from build123d import *

# Parameters (mm, degrees)
EXTRUDE_1_DEPTH     = 3
SKETCH_2_W          = 10.5
SKETCH_2_H          = 3.5
CUT_EXTRUDE_1_DEPTH = 150.258104234


with BuildPart() as part:
    # Эскиз1 → Бобышка-Вытянуть1 (new body)
    with BuildSketch(Plane(origin=(0, 0, 0), x_dir=(1, 0, 0), z_dir=(0, 1, 0))):
        with BuildLine():
            Line((-135, -31.788922156), (-138, -31.788922156))
            Line((-138, -31.788922156), (-138, -21.788922156))
            Line((-138, -21.788922156), (-135, -21.788922156))
            Line((-135, -21.788922156), (-135, -16.788922156))
            Line((-135, -16.788922156), (-138, -16.788922156))
            Line((-138, -16.788922156), (-138, -6.788922156))
            Line((-138, -6.788922156), (-135, -6.788922156))
            Line((-135, -6.788922156), (-135, 3.211077844))
            Line((-135, 3.211077844), (-125, 3.211077844))
            Line((-125, 3.211077844), (75, 3.211077844))
            Line((75, 3.211077844), (85, 3.211077844))
            Line((85, 3.211077844), (85, -6.788922156))
            Line((85, -6.788922156), (88, -6.788922156))
            Line((88, -6.788922156), (88, -16.788922156))
            Line((88, -16.788922156), (85, -16.788922156))
            Line((85, -16.788922156), (85, -21.788922156))
            Line((85, -21.788922156), (88, -21.788922156))
            Line((88, -21.788922156), (88, -31.788922156))
            Line((88, -31.788922156), (85, -31.788922156))
            Line((85, -31.788922156), (85, -36.788922156))
            Line((85, -36.788922156), (88, -36.788922156))
            Line((88, -36.788922156), (88, -46.788922156))
            Line((88, -46.788922156), (85, -46.788922156))
            Line((85, -46.788922156), (85, -56.788922156))
            Line((85, -56.788922156), (55, -56.788922156))
            Line((55, -56.788922156), (55, -26.788922156))
            ThreePointArc((55, -26.788922156), (52.071067812, -19.717854344), (45, -16.788922156))
            Line((45, -16.788922156), (-95, -16.788922156))
            ThreePointArc((-95, -16.788922156), (-102.071067812, -19.717854344), (-105, -26.788922156))
            Line((-105, -26.788922156), (-105, -56.788922156))
            Line((-105, -56.788922156), (-135, -56.788922156))
            Line((-135, -56.788922156), (-135, -46.788922156))
            Line((-135, -46.788922156), (-138, -46.788922156))
            Line((-138, -46.788922156), (-138, -36.788922156))
            Line((-138, -36.788922156), (-135, -36.788922156))
            Line((-135, -36.788922156), (-135, -31.788922156))
        make_face()
    extrude(amount=EXTRUDE_1_DEPTH)

    # Эскиз2 → Вырез-Вытянуть1 (cut, through all)
    with BuildSketch(Plane(origin=(0, 0, 0), x_dir=(1, 0, 0), z_dir=(0, 1, 0))):
        with Locations((-115, -10.788922156)):
            Rectangle(SKETCH_2_W, SKETCH_2_H)
        with Locations((-95, -10.788922156)):
            Rectangle(SKETCH_2_W, SKETCH_2_H)
        with Locations((-75, -10.788922156)):
            Rectangle(SKETCH_2_W, SKETCH_2_H)
        with Locations((-55, -10.788922156)):
            Rectangle(SKETCH_2_W, SKETCH_2_H)
        with Locations((-35, -10.788922156)):
            Rectangle(SKETCH_2_W, SKETCH_2_H)
        with Locations((-15, -10.788922156)):
            Rectangle(SKETCH_2_W, SKETCH_2_H)
        with Locations((5, -10.788922156)):
            Rectangle(SKETCH_2_W, SKETCH_2_H)
        with Locations((25, -10.788922156)):
            Rectangle(SKETCH_2_W, SKETCH_2_H)
        with Locations((45, -10.788922156)):
            Rectangle(SKETCH_2_W, SKETCH_2_H)
        with Locations((65, -10.788922156)):
            Rectangle(SKETCH_2_W, SKETCH_2_H)
    extrude(amount=CUT_EXTRUDE_1_DEPTH, mode=Mode.SUBTRACT)


solid = part.part
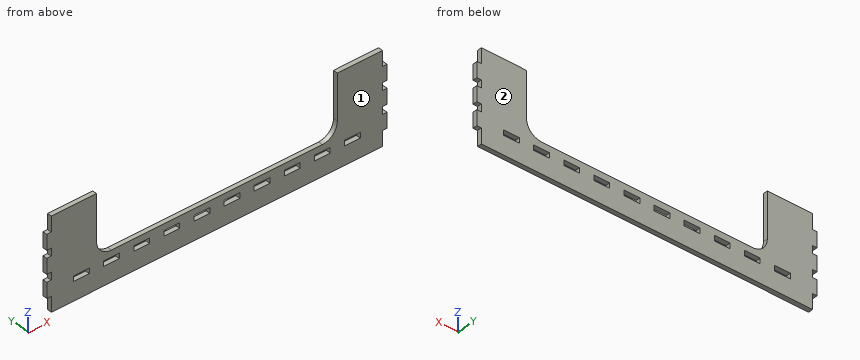
Work out the finished part from the listing and answer in its coordinate system (mm). Face numbers are marked on the shaded views. Give positions to 0.01 mm unless a question says otherwise; leave off trailing zeros. Loops run counter-clockwise (first coordinate to the right, second up) from the corner with the lowest first, then second, coordinate; pieces in that order, holes last. Notation, with made-up numbers: (47, 51) -> (72, 51) arc R25 cw to (72, 74) -> close; hole circle Ø5 at (24, 15). An arc over 180 degrees is marked (long way). Use a Markdown table: item, result. Add a question column.
1. Find the intervals of material crossed by probe 1 along Z at (x, y) = (5.5, 2.1); probe 2 along Z at (x, y) = (62, 0.45); probe 3 along X at (y, z) = (2.25, 38), in increasing order.
2. Section A-A on x = -117 is taken. Determine the outline of the cut face in (y, z), and give its area (4 significant figures).
3. Section C-C on y = 2.2 is taken. State how many separate pieces and enclosed holes the cut face has, and give its area (3 significant figures).
4. Determine the mould class of the marked faces 1 and 2 for opening direction Y: released by +Y, released by -Y, zero draft, split by the parting line, or undercut.
5. Section B-B on z = 39.5 is taken. Determine the outline of the cut face in (x, y).
6. Flat-ended cylindrical pins translate along their axes: pin 1 Ø1 at (x, y) = (36.5, 2) entering from +Z; pin 2 Ø0.9 at (x, y) = (87, 1) entering from -Z. Find the tip coordinate at first contact, or state that the pin passes through.
Results below:
| question | item | result |
|---|---|---|
| 1 | probe 1 | z = -3.21 to 9.04, 12.54 to 16.79 |
| 1 | probe 2 | z = -3.21 to 9.04, 12.54 to 56.79 |
| 1 | probe 3 | x = -138 to -105, 55 to 88 |
| 2 | outline | (0, -3.21) -> (3, -3.21) -> (3, 9.04) -> (0, 9.04) -> close; (0, 12.54) -> (3, 12.54) -> (3, 56.79) -> (0, 56.79) -> close |
| 2 | area | 169.5 mm^2 |
| 3 | separate pieces | 1 |
| 3 | enclosed holes | 10 |
| 3 | area | 6,660 mm^2 |
| 4 | face 1 | released by -Y |
| 4 | face 2 | released by +Y |
| 5 | outline | (-138, 0) -> (-105, 0) -> (-105, 3) -> (-138, 3) -> close; (55, 0) -> (88, 0) -> (88, 3) -> (55, 3) -> close |
| 6 | pin 1 | stops at z = 16.79 |
| 6 | pin 2 | stops at z = 6.79 |
